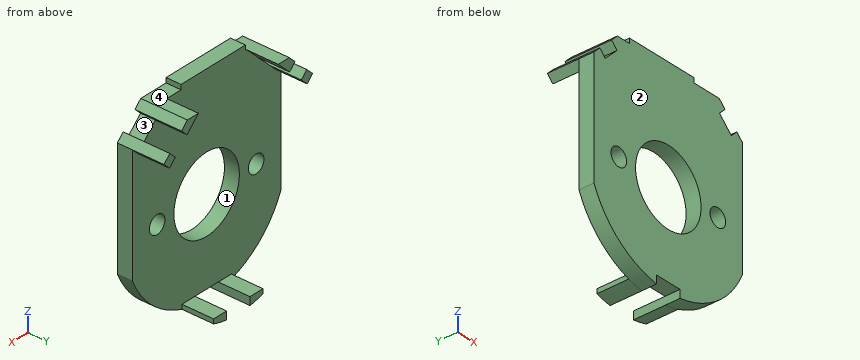
from build123d import *

# Parameters (mm, degrees)
SKETCH1_R               = 1.5
SKETCH1_R_2             = 6.3
BOSS_EXTRUDE1_DEPTH     = 2.5
CUT_EXTRUDE1_DEPTH      = 24.681302751
CUT_EXTRUDE1_DEPTH_BACK = 24.681302751
BOSS_EXTRUDE2_DEPTH     = 5.3


with BuildPart() as part:
    # Sketch1 → Boss-Extrude1 (new body)
    with BuildSketch(Plane(origin=(0, 0, 0), x_dir=(1, 0, 0), z_dir=(0, 1, 0))):
        with BuildLine():
            Line((-14.3, 6.139966555), (-14.3, -13.41))
            Line((-14.3, -13.41), (-9.8, -17.91))
            Line((-9.8, -17.91), (-7.47, -17.91))
            Line((-7.47, -17.91), (-7.47, -18.71))
            Line((-7.47, -18.71), (4.92, -18.71))
            Line((4.92, -18.71), (4.92, -17.91))
            Line((4.92, -17.91), (9.8, -17.91))
            Line((9.8, -17.91), (14.3, -13.41))
            Line((14.3, -13.41), (14.3, 6.139966555))
            ThreePointArc((14.3, 6.139966555), (9.505716305, 12.4030126), (2.25, 15.495824073))
            Line((2.25, 15.495824073), (2.25, 14.16))
            Line((2.25, 14.16), (-2.25, 14.16))
            Line((-2.25, 14.16), (-2.25, 15.495824073))
            ThreePointArc((-2.25, 15.495824073), (-9.505716305, 12.4030126), (-14.3, 6.139966555))
        make_face()
        with Locations(Location((9.525, 0, 0), (0, 0, 270))):
            Circle(SKETCH1_R, mode=Mode.SUBTRACT)
        with Locations(Location((-9.525, 0, 0), (0, 0, 90))):
            Circle(SKETCH1_R, mode=Mode.SUBTRACT)
        with Locations(Location((0, 0, 0), (0, 0, 270))):
            Circle(SKETCH1_R_2, mode=Mode.SUBTRACT)
    extrude(amount=BOSS_EXTRUDE1_DEPTH)

    # Sketch2 → Cut-Extrude1 (cut, two sides: drawn at the far end of the back side and taken through both)
    with BuildSketch(Plane(origin=(0, 2.5, 0), x_dir=(1, 0, 0), z_dir=(0, 1, 0)).offset(-CUT_EXTRUDE1_DEPTH_BACK)):
        Polygon((-12.120710678, -13.467968978), (-9.857968978, -15.730710678), (-10.91862915, -16.79137085), (-13.18137085, -14.52862915), align=None)
        Polygon((12.120710678, -13.467968978), (13.18137085, -14.52862915), (10.91862915, -16.79137085), (9.857968978, -15.730710678), align=None)
    extrude(amount=CUT_EXTRUDE1_DEPTH + CUT_EXTRUDE1_DEPTH_BACK, mode=Mode.SUBTRACT)

    # Sketch3 → Boss-Extrude2 (add)
    with BuildSketch(Plane(origin=(0, 2.5, 0), x_dir=(1, 0, 0), z_dir=(0, 1, 0))):
        Polygon((-13.18137085, -14.52862915), (-14.3, -13.41), (-13.239339828, -12.349339828), (-12.120710678, -13.467968978), align=None)
        Polygon((-10.91862915, -16.79137085), (-9.857968978, -15.730710678), (-7.678679656, -17.91), (-9.8, -17.91), align=None)
        Polygon((13.239339828, -12.349339828), (12.120710678, -13.467968978), (13.18137085, -14.52862915), (14.3, -13.41), align=None)
        Polygon((7.678679656, -17.91), (9.8, -17.91), (10.91862915, -16.79137085), (9.857968978, -15.730710678), align=None)
        with BuildLine():
            Line((2.25, 15.495824073), (2.25, 14.16))
            Line((2.25, 14.16), (4.75, 14.16))
            Line((4.75, 14.16), (4.75, 14.91423668))
            ThreePointArc((4.75, 14.91423668), (3.512059364, 15.256868517), (2.25, 15.495824073))
        make_face()
        with BuildLine():
            Line((-2.25, 15.495824073), (-2.25, 14.16))
            Line((-2.25, 14.16), (-4.75, 14.16))
            Line((-4.75, 14.16), (-4.75, 14.91423668))
            ThreePointArc((-4.75, 14.91423668), (-3.512059364, 15.256868517), (-2.25, 15.495824073))
        make_face()
    extrude(amount=BOSS_EXTRUDE2_DEPTH)


solid = part.part
Could you check a few things on this model? Use its own coordinates, in mm. Face numbers are marked on the shaded views. A direction names the side the tool comes from. Round coordinates to 2 decimals unless told otherwise and drop trailing zeros. Loops run counter-clockwise (first coordinate to the right, second up) from the corner with the lowest first, then second, coordinate; pieces in that order, holes last. Notation, with made-up numbers: (21, -34.5) - (71, -34.5) arc R23 ccw to (71, -25.5) - close; hole circle Ø9 at (59, 22.25). An arc over 180 degrees is marked (long way). Write item = value, one per line.
1) On a 3-axis mill with a long thin cutter (end or side, diameter ignored), from which of +Z, -Z, +X, -X, +Y, -Y can I reach the whole of each face in a straight line? I mean the marked faces 3 and 4. Say none if no direction works.
Computed:
face_3 = +Y, -Y
face_4 = +Z, +X, +Y, -Y
2) Imagine slicing it at A-A (y = 5.5). Please give me the cut outline in (x, z).
Computed:
outline = (-14.3, 13.41) - (-13.24, 12.35) - (-12.12, 13.47) - (-13.18, 14.53) - close; (-10.92, 16.79) - (-9.86, 15.73) - (-7.68, 17.91) - (-9.8, 17.91) - close; (-4.75, -14.91) arc R15.5 ccw to (-2.25, -15.5) - (-2.25, -14.16) - (-4.75, -14.16) - close; (2.25, -15.5) arc R15.5 ccw to (4.75, -14.91) - (4.75, -14.16) - (2.25, -14.16) - close; (7.68, 17.91) - (9.86, 15.73) - (10.92, 16.79) - (9.8, 17.91) - close; (12.12, 13.47) - (13.24, 12.35) - (14.3, 13.41) - (13.18, 14.53) - close
3) Imagine slicing it at D-D (y = 1.75). Please give me the cut outline in (x, z) (3 decimals).
Computed:
outline = (-14.3, -6.14) arc R15.5 ccw to (-2.25, -15.496) - (-2.25, -14.16) - (2.25, -14.16) - (2.25, -15.496) arc R15.5 ccw to (14.3, -6.14) - (14.3, 13.41) - (13.181, 14.529) - (12.121, 13.468) - (9.858, 15.731) - (10.919, 16.791) - (9.8, 17.91) - (4.92, 17.91) - (4.92, 18.71) - (-7.47, 18.71) - (-7.47, 17.91) - (-9.8, 17.91) - (-10.919, 16.791) - (-9.858, 15.731) - (-12.121, 13.468) - (-13.181, 14.529) - (-14.3, 13.41) - close; hole circle Ø3 at (-9.525, 0); hole circle Ø12.6 at (0, 0); hole circle Ø3 at (9.525, 0)
4) Imagine slicing it at B-B (x = 0). Please give me the cut outline in (y, z).
Computed:
outline = (0, -14.16) - (2.5, -14.16) - (2.5, -6.3) - (0, -6.3) - close; (0, 6.3) - (2.5, 6.3) - (2.5, 18.71) - (0, 18.71) - close
5) If we mould it in two halves opening along X, with no side actions, what happens to the marked faces 1 and 2? For each: pulls with the +X half, pulls with the -X half, needs draft (parallel to the pull), parting line crosses it, or undercut.
Computed:
face_1 = undercut
face_2 = needs draft
6) I need wall thicknesses on line 1 along X through (y, z) = (1.8, 0) (3 decimals); line 2 along Y through (x, z) = (8, -3.5); line 3 along Z through (x, y) = (-5.5, 1). Which ranges of each line are inside material? Lowest first, please. Write a range as from..to.
Computed:
line_1 = -14.3..-11.025, -8.025..-6.3, 6.3..8.025, 11.025..14.3
line_2 = 0..2.5
line_3 = -14.65..-3.07, 3.07..18.71
7) Imagine slicing it at C-C (z = 0). Please give me the cut outline in (x, y) (3 decimals).
Computed:
outline = (-14.3, 0) - (-11.025, 0) - (-11.025, 2.5) - (-14.3, 2.5) - close; (-8.025, 0) - (-6.3, 0) - (-6.3, 2.5) - (-8.025, 2.5) - close; (6.3, 0) - (8.025, 0) - (8.025, 2.5) - (6.3, 2.5) - close; (11.025, 0) - (14.3, 0) - (14.3, 2.5) - (11.025, 2.5) - close
8) I'm going to push flat-ended pins straight in: P1, Ø0.8, axis at y = 5.5, z = -14.5, coming from the -X side; P2, Ø1.1, axis at y = 4.5, z = -15, coming from the +X side; P3, Ø3, axis at y = 1.5, z = -10.5, coming from the +X side; P4, Ø11.5, axis at x = 0, z = 0, coming from the +Y side. Where does each tip first touch, or does it pass through?
Computed:
P1 = -4.75
P2 = 4.75
P3 = 12.73
P4 = through
